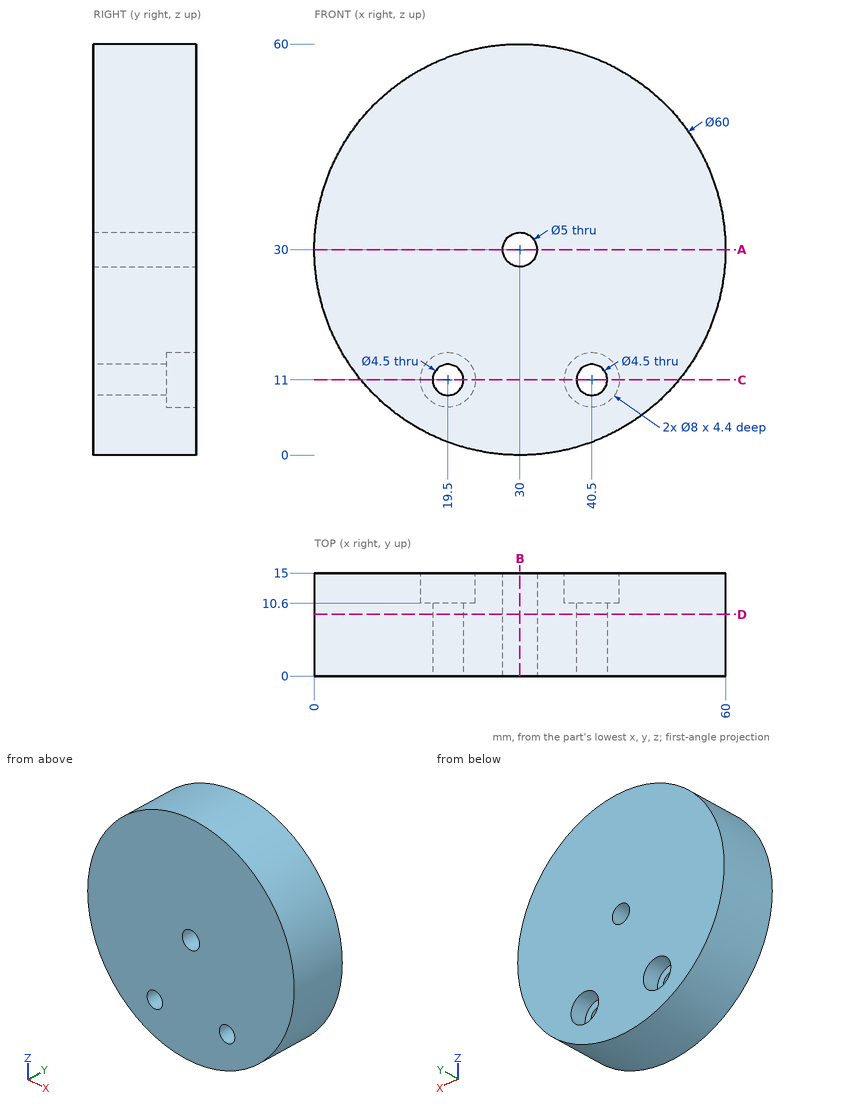
Print and shaded views of the part. All mm, measured from the part's lowest x, y and z. Coordinates: 2 decimals unless noted, no trailing zeros. Order: outer loops, then holes, each group sorted by start corner. A loop starts at its lowest first (then second) coordinate and runs counter-clockwise, first axis right, second up.
Item 1: Saw through at C-C on z = 11. List the corners of the cut face in (x, y), then the cut area to 3 significant figures.
Filled in:
outline: (6.78, 0) - (17.25, 0) - (17.25, 10.6) - (15.5, 10.6) - (15.5, 15) - (6.78, 15) - close; (21.75, 0) - (38.25, 0) - (38.25, 10.6) - (36.5, 10.6) - (36.5, 15) - (23.5, 15) - (23.5, 10.6) - (21.75, 10.6) - close; (42.75, 0) - (53.22, 0) - (53.22, 15) - (44.5, 15) - (44.5, 10.6) - (42.75, 10.6) - close
area: 531 mm2
Item 2: Saw through at A-A on z = 30. List the corners of the cut face in (x, y).
Filled in:
outline: (0, 0) - (27.5, 0) - (27.5, 15) - (0, 15) - close; (32.5, 0) - (60, 0) - (60, 15) - (32.5, 15) - close
Item 3: Saw through at B-B on x = 30. List the corners of the cut face in (y, z), then the cut area to 3 significant figures.
Filled in:
outline: (0, 0) - (15, 0) - (15, 27.5) - (0, 27.5) - close; (0, 32.5) - (15, 32.5) - (15, 60) - (0, 60) - close
area: 825 mm2
Item 4: Saw through at D-D on y = 9. List the corners of the cut face in (x, z), then the cut area to 3 significant figures.
Filled in:
outline: circle Ø60 at (30, 30); hole circle Ø4.5 at (19.5, 11); hole circle Ø5 at (30, 30); hole circle Ø4.5 at (40.5, 11)
area: 2,780 mm2
Item 5: Drill centre lines: L1, parallel to Z at x = 30, y = 7.75; L2, parallel to X at y = 4.75, z = 11; L3, parallel to Z at x = 31, y = 13.75. Where is each one in solid material? Low to high.
Filled in:
L1: z = 0 to 27.5, 32.5 to 60
L2: x = 6.78 to 17.25, 21.75 to 38.25, 42.75 to 53.22
L3: z = 0.02 to 27.71, 32.29 to 59.98
Item 6: Drop flat-ended pins along their axis: pin 1 Ø1.5 at (x, y) = (19.5, 8.5) entering from +Z; pin 2 Ø10.5 at (x, z) = (19.5, 11) entering from -Y; pin 3 Ø1 at (y, z) = (10, 12.5) entering from +X; pin 4 Ø4 at (x, z) = (19.5, 11) entering from +Y. Give the stop position or say it passes through.
Filled in:
pin 1: stops at z = 58.37
pin 2: stops at y = 0
pin 3: stops at x = 54.72
pin 4: passes through
